Autodesk Inventor part; units mm, degrees
ref_plane "YZ Plane" through (0, 0, 0) normal (1, 0, 0) x (0, 1, 0)
ref_plane "XZ Plane" through (0, 0, 0) normal (0, 1, 0) x (-1, 0, 0)
ref_plane "XY Plane" through (0, 0, 0) normal (0, 0, 1) x (1, 0, 0)
sketch "Sketch1" plane through (0, 0, 0) normal (0, 0, 1) x (1, 0, 0)
  point P0 (0, 0)
ref_plane "Work Plane1" through (0, 0, 0) normal (0, 0, 1) x (1, 0, 0)
sketch "Sketch5" plane through (0, 0, 0) normal (0, 0, 1) x (1, 0, 0)
  circle A0 centre (-15.5, 0) radius 1.5
  circle A1 centre (0, 0) radius 18.4
  line L0 (-18.4, 0) -> (18.4, 0)
  line L1 (-1.5961, -18.3306) -> (-1.5961, -18.3306)
  line L2 (0, 18.4) -> (0, -18.4)
  circle A2 centre (0, -7) radius 6
  circle A3 centre (15.5, 0) radius 1.5
  circle A4 centre (0, 0) radius 15.5
  line L3 (-11.863, 20.6629) -> (9.25, -15.9059)
  circle A5 centre (0, 0) radius 18.4
  line L4 (-9.2, -15.9349) -> (9.2, 15.9349)
  circle A6 centre (7.8, -13.3944) radius 1.5
  circle A7 centre (7.75, 13.4234) radius 1.5
  circle A8 centre (-7.75, -13.4234) radius 1.5
  circle A9 centre (-7.6999, 13.4522) radius 1.5
  line L5 (0, 0) -> (-21.575, 0)
  line L6 (-21.575, 0) -> (-21.575, 21.575)
  line L7 (-21.575, 21.575) -> (21.575, 21.575)
  line L8 (21.575, 21.575) -> (21.575, -30.3062)
  line L9 (21.575, -30.3062) -> (-21.575, -30.3062)
  line L10 (-21.575, -30.3062) -> (-21.575, 21.575)
  point P0 (7.75, 13.4234)
  point P1 (7.8, -13.3944)
  point P2 (-0.5944, -1.0295)
  point P3 (0, 0.1156)
  point P4 (0.6654, -1.037)
  point P5 (0.0667, 0)
  dimension "d10" = 3
  dimension "d11" = 12
  dimension "d12" = 7
  dimension "d15" = 3
  dimension "d16" = 31
  dimension "d17" = 2.9
  dimension "d19" = 60
  dimension "d20" = 60
  dimension "d21" = 3
  dimension "d22" = 3
  dimension "d23" = 3
  dimension "d24" = 3
  dimension "d33" = 21.575
  dimension "d34" = 43.15
  dimension "d35" = 30.3062
  dimension "d36" = 21.575
extrude "Extrusion8" add sketch "Sketch5" along normal blind 6.35 contours L0 L4 A2 A8 A4 A0 | A0 A4 A9 L3 L2 L0 | A0 L0 A1 L3 A9 A4 | A4 A8 L4 A1 L0 A0 | L0 L3 A2 L2 | L2 A2 L4 | L3 L4 A7 A4 A3 L0 | L0 A3 A4 A6 L3 A2 | L3 A9 A4 L2 | L2 A4 A7 L4 L3 | L6 L7 L8 L9 L10 | L3 A1 L2 A4 A9 | L4 A2 L2 A4 A8 | A8 A4 L2 A1 L4 | L2 A1 L4 A7 A4 | A2 L3 A6 A4 L2 | A4 A7 L4 A1 L0 A3 | A3 L0 A1 L3 A6 A4 | A4 A6 L3 A1 L2 picked at (-0.0661, -0.6678)
equation "\"d33\" = MountOffset"
equation "\"d34\" = 2 * MountOffset"
equation "\"d37\" = mountDepth"
equation "\"motorDiameter\" = 36.8"
equation "\"mountDepth\" = 6.35"
properties part number "Motor"
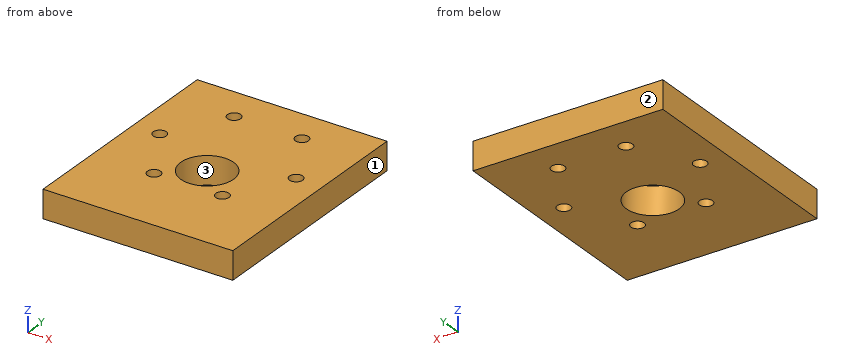
Work out the finished part from the listing and answer in its coordinate system (mm). Face numbers are marked on the shaded views. Coordinates: 2 decimals unless noted, no trailing zeros. Order: outer loops, then holes, each group sorted by start corner. A loop starts at its lowest first (then second) coordinate and runs counter-clockwise, first axis right, second up. Notation, with made-up numbers: (0, -32.5) - (21, -32.5) arc R27 cw to (21, 2.5) - close; hole circle Ø8 at (37, 19.25). An arc over 180 degrees is marked (long way). Put each result on its own line as item: value. Start each with the question number.
1) Find the intervals of material crossed by line 1 (Y direction, x = 7.8, z = 3.75) (3 decimals); line 2 (X direction, y = -7, z = 3.75) (3 decimals); line 3 (Y direction, x = -15.5, z = 4.25) (3 decimals), in increasing order. Write a range as from..to.
2) Find section D-D (z = 3.25). State how many separate pieces and enclosed holes the cut face has, plus the area to 3 significant figures.
3) Find section A-A (x = -15.5). Give the vertices of the cut face in (y, z) (3 decimals).
4) A flat-ended cylindrical pin translates along its axis: pin 1 (1.8 mm diameter, centred on x = -15.5, y = 0, fed in from +Z). Find the tip coordinate at first contact, or state that the pin passes through.
5) For a pull along X with two mould halves and no side action, classify the marked faces 1, 2 and 3 as released by +X, released by -X, zero draft, split by the parting line, or undercut.
6) Find section C-C (x = 7.75). Give the vertices of the cut face in (y, z) (3 decimals).
7) Find section B-B (y = -10.5). Give the vertices of the cut face in (x, z) (3 decimals).
Results list:
1. line 1: y = -30.306..-14.894, -11.894..11.924, 14.923..21.575
1. line 2: x = -21.575..-6, 6..21.575
1. line 3: y = -30.306..-1.5, 1.5..21.575
2. separate pieces: 1
2. enclosed holes: 8
2. area: 2,080 mm^2
3. outline: (-30.306, 0) - (-1.5, 0) - (-1.5, 6.35) - (-30.306, 6.35) - close; (1.5, 0) - (21.575, 0) - (21.575, 6.35) - (1.5, 6.35) - close
4. pin 1: passes through
5. face 1: released by +X
5. face 2: zero draft
5. face 3: undercut
6. outline: (-30.306, 0) - (-14.894, 0) - (-14.894, 6.35) - (-30.306, 6.35) - close; (-11.895, 0) - (11.923, 0) - (11.923, 6.35) - (-11.895, 6.35) - close; (14.923, 0) - (21.575, 0) - (21.575, 6.35) - (14.923, 6.35) - close
7. outline: (-21.575, 0) - (-4.873, 0) - (-4.873, 6.35) - (-21.575, 6.35) - close; (4.873, 0) - (21.575, 0) - (21.575, 6.35) - (4.873, 6.35) - close
